from build123d import *

# Parameters (mm, degrees)
F2_R     = 3.175
F3_DEPTH = 6.35
F5_DEPTH = 0.0635


with BuildPart() as f1:
    # F0 (on Front) → F1 (revolve)
    with BuildSketch(Plane.XZ):
        with BuildLine():
            Line((-30.074457, 23.07059), (-30.074457, 28.78559))
            Line((-30.074457, 28.78559), (-36.424457, 28.78559))
            ThreePointArc((-36.424457, 28.78559), (-38.996207, 25.92809), (-36.424457, 23.07059))
            Line((-36.424457, 23.07059), (-30.074457, 23.07059))
        make_face()
    revolve(axis=Axis((-30.074457, 0, 26.24559), (0, 0, -1)))

    # F2 (on face) → F3 (join)
    with BuildSketch(Plane(origin=(0, 0, 23.07059), x_dir=(1, 0, 0), z_dir=(0, 0, -1))):
        with Locations((-30.074457, 0)):
            Circle(F2_R)
    extrude(amount=F3_DEPTH)

    # F4 (on face) → F5 (join)
    with BuildSketch(Plane(origin=(0, 0, 16.72059), x_dir=(1, 0, 0), z_dir=(0, 0, -1))):
        Polygon((-30.765451, -0.924808), (-29.620068, -1.065534), (-29.620068, 1.96214), (-30.765451, 1.96214), align=None)
        Polygon((-30.765451, -1.246022), (-29.620068, -1.246022), (-29.620068, -1.065534), (-30.765451, -0.924808), align=None)
        Polygon((-29.620068, -1.065534), (-29.620068, -1.246022), (-30.765451, -1.246022), (-30.765451, -0.924808), (-31.044574, -0.890514), (-30.381126, -2.453838), (-29.358972, -1.097613), align=None)
    extrude(amount=F5_DEPTH)


solid = f1.part
The listing builds one solid part. Answer for the finished solid, in the listing's coordinates (mm). A direction names the side the tool comes from. Coordinates: 2 decimals unless noted, no trailing zeros. Loops run counter-clockwise (first coordinate to the right, second up) from the corner with the lowest first, then second, coordinate; pieces in that order, holes last.
1) Find the intervals of material crossed by L1, parallel to Z at x = -26.75, y = 4.75; L2, parallel to Z at x = -32.25, y = -1.5; L3, parallel to X at y = -0.5, z = 22.5, in increasing order.
2) Find section A-A on y = 0. Write down the section's boundary in (x, z).
3) A tool of negligible diameter and unlimited length cuts with its end or side. For faces 1 (the face through (-27, 2, 23.071)), 2 (the face through (-30, 0, 28.786)), from which of +Z, -Z, +X, -X, +Y, -Y can it reach the whole face along a straight path? Write none if from no direction.
4) Flat-ended cylindrical pins translate along their axes: pin 1 Ø1.5 at (y, z) = (-1.5, 27) entering from -X; pin 2 Ø4 at (x, z) = (-31.5, 22.5) entering from -Y; pin 3 Ø2 at (x, z) = (-29, 18.5) entering from +Y; pin 4 Ø1 at (x, z) = (-23.5, 21.5) entering from -Y. Find the tip coordinate at first contact, or state that the pin passes through.
5) Find section B-B on z = 20.25. Write down the section's boundary in (x, y) (3 decimals), then the cut area to 3 significant figures.
6) Find section C-C on z = 26.75. Write down the section's boundary in (x, y).
Values:
1. L1: z = 23.07 to 28.79
1. L2: z = 16.72 to 28.79
1. L3: x = -33.21 to -26.94
2. outline: (-36.42, 23.07) - (-33.25, 23.07) - (-33.25, 16.72) - (-30.77, 16.72) - (-30.77, 16.66) - (-29.62, 16.66) - (-29.62, 16.72) - (-26.9, 16.72) - (-26.9, 23.07) - (-23.72, 23.07) arc R2.87 ccw to (-23.72, 28.79) - (-36.42, 28.79) arc R2.87 ccw to start
3. face 1: -Z
3. face 2: +Z, +X, -X, +Y, -Y
4. pin 1: stops at x = -38.89
4. pin 2: stops at y = -8.46
4. pin 3: stops at y = 3.17
4. pin 4: passes through
5. outline: circle Ø6.35 at (-30.074, 0)
5. area: 31.7 mm2
6. outline: circle Ø17.6 at (-30.07, 0)
